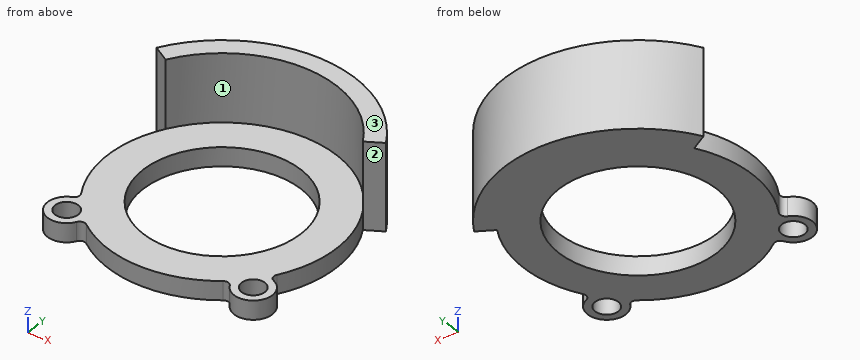
from build123d import *

# Parameters (mm, degrees)
ESBO_O1_R                = 21
ESBO_O1_R_2              = 3.1
RESSALTO_EXTRUS_O1_DEPTH = 5
RESSALTO_EXTRUS_O2_DEPTH = 18


with BuildPart() as part:
    # Esboço1 → Ressalto-extrusão1 (new body)
    with BuildSketch(Plane.XY):
        with BuildLine():
            Line((-26.413774815, 15.25), (-30.743901834, 17.75))
            ThreePointArc((-30.743901834, 17.75), (0, 35.5), (30.743901834, 17.75))
            Line((30.743901834, 17.75), (26.413774815, 15.25))
            ThreePointArc((26.413774815, 15.25), (30.49940407, -0.19066032), (26.22105388, -15.579035061))
            ThreePointArc((26.22105388, -15.579035061), (26.087819075, -16.82024855), (26.940019837, -17.73245264))
            ThreePointArc((26.940019837, -17.73245264), (28.794642857, -25.856499042), (20.518582449, -24.883575301))
            ThreePointArc((20.518582449, -24.883575301), (19.520268693, -24.134087419), (18.30049416, -24.399629372))
            ThreePointArc((18.30049416, -24.399629372), (0, -30.5), (-18.30049416, -24.399629372))
            ThreePointArc((-18.30049416, -24.399629372), (-19.520268693, -24.134087419), (-20.518582449, -24.883575301))
            ThreePointArc((-20.518582449, -24.883575301), (-28.794642857, -25.856499042), (-26.940019837, -17.73245264))
            ThreePointArc((-26.940019837, -17.73245264), (-26.087819075, -16.82024855), (-26.22105388, -15.579035061))
            ThreePointArc((-26.22105388, -15.579035061), (-30.49940407, -0.19066032), (-26.413774815, 15.25))
        make_face()
        Circle(ESBO_O1_R, mode=Mode.SUBTRACT)
        with Locations((25, -22.449053432)):
            Circle(ESBO_O1_R_2, mode=Mode.SUBTRACT)
        with Locations((-25, -22.449053432)):
            Circle(ESBO_O1_R_2, mode=Mode.SUBTRACT)
    extrude(amount=RESSALTO_EXTRUS_O1_DEPTH)

    # Esboço2 → Ressalto-extrusão2 (add)
    with BuildSketch(Plane.XY.offset(5)):
        with BuildLine():
            Line((-26.413774815, 15.25), (-30.743901834, 17.75))
            ThreePointArc((-30.743901834, 17.75), (0, 35.5), (30.743901834, 17.75))
            Line((30.743901834, 17.75), (26.413774815, 15.25))
            ThreePointArc((26.413774815, 15.25), (0, 30.5), (-26.413774815, 15.25))
        make_face()
    extrude(amount=RESSALTO_EXTRUS_O2_DEPTH)


solid = part.part
Here's how the part is built. I have some questions about the finished solid (model axes, mm). Face numbers are marked on the shaded views. A direction names the side the tool comes from. Coordinates: 2 decimals unless noted, no trailing zeros. Order: outer loops, then holes, each group sorted by start corner. A loop starts at its lowest first (then second) coordinate and runs counter-clockwise, first axis right, second up. Notation, with made-up numbers: (-21, 18) -> (-16, 18) arc R30 ccw to (-16, 54) -> close; hole circle Ø8 at (9.5, 60.25). An arc over 180 degrees is marked (long way). Answer in a Markdown table with one row per item.
(1) I want a section at D-D on x = -25. List the corners of the cut face in (y, z) for me.
Answer key:
| item | result |
|---|---|
| outline | (-27.55, 0) -> (-25.55, 0) -> (-25.55, 5) -> (-27.55, 5) -> close; (-19.35, 0) -> (25.2, 0) -> (25.2, 23) -> (17.47, 23) -> (17.47, 5) -> (-19.35, 5) -> close |
(2) I want a section at C-C on y = 27. List the corners of the cut face in (x, z) for me, then the cut area to 3 significant figures.
Answer key:
| item | result |
|---|---|
| outline | (-23.05, 0) -> (23.05, 0) -> (23.05, 23) -> (14.19, 23) -> (14.19, 5) -> (-14.19, 5) -> (-14.19, 23) -> (-23.05, 23) -> close |
| area | 550 mm^2 |
(3) On a 3-axis mill with a long thin cutter (end or side, diameter ignored), from which of +Z, -Z, +X, -X, +Y, -Y can I reach the whole of each face in a straight line? I mean the marked faces 1, 2 and 3. Say none if no direction works.
Answer key:
| item | result |
|---|---|
| face 1 | +Z, -Y |
| face 2 | +Z, -Z, +X |
| face 3 | +Z, +X, -X, +Y, -Y |
(4) I want a section at A-A on x = 0. List the corners of the cut face in (y, z) for me, then the cut area to 3 significant figures.
Answer key:
| item | result |
|---|---|
| outline | (-30.5, 0) -> (-21, 0) -> (-21, 5) -> (-30.5, 5) -> close; (21, 0) -> (35.5, 0) -> (35.5, 23) -> (30.5, 23) -> (30.5, 5) -> (21, 5) -> close |
| area | 210 mm^2 |
(5) Will these pins go through, and if not, where does the flat tip stop? pin 1 Ø7 at (x, y) = (-25, -22.45) entering from +Z; pin 2 Ø6 at (x, z) = (18, 6.5) entering from -Y; pin 3 Ø2 at (x, z) = (-8, 14.5) entering from -Y; pin 4 Ø3.5 at (x, y) = (25, -22.45) entering from -Z.
Answer key:
| item | result |
|---|---|
| pin 1 | z = 5 |
| pin 2 | y = -26.33 |
| pin 3 | y = 29.14 |
| pin 4 | through |
(6) I want a section at B-B on z = 3. List the corners of the cut face in (x, y) for me, then the cut area to 3 significant figures.
Answer key:
| item | result |
|---|---|
| outline | (-30.74, 17.75) -> (-26.41, 15.25) arc R30.5 ccw to (-26.22, -15.58) arc R1.5 cw to (-26.94, -17.73) arc R5.1 ccw (long way) to (-20.52, -24.88) arc R1.5 cw to (-18.3, -24.4) arc R30.5 ccw to (18.3, -24.4) arc R1.5 cw to (20.52, -24.88) arc R5.1 ccw (long way) to (26.94, -17.73) arc R1.5 cw to (26.22, -15.58) arc R30.5 ccw to (26.41, 15.25) -> (30.74, 17.75) arc R35.5 ccw to start; hole circle Ø6.2 at (-25, -22.45); hole circle Ø42 at (0, 0); hole circle Ø6.2 at (25, -22.45) |
| area | 1,970 mm^2 |
(7) Please list where these lines run through material, in increasing order: probe 1 along Z at (x, y) = (25.5, 3); probe 2 along X at (y, z) = (15.5, 9.5); probe 3 along X at (y, z) = (22.5, 10).
Answer key:
| item | result |
|---|---|
| probe 1 | 0 to 5 |
| probe 2 | -26.85 to -26.27, 26.27 to 26.85 |
| probe 3 | -27.46 to -20.59, 20.59 to 27.46 |
